Autodesk Inventor part; units mm, degrees
ref_plane "Work Plane1" through (-2.8393, 0, 0) normal (0, 0, -1) x (-1, 0, 0)
ref_plane "Work Plane2" through (0, 0, 4.58) normal (1, 0, 0) x (0, 0, -1)
ref_plane "Work Plane3" through (0, 45, 0) normal (0, 1, 0) x (1, 0, 0)
sketch "Sketch1" plane through (0, 0, 0) normal (0, 1, 0) x (-1, 0, 0)
  circle A0 centre (0, 0) radius 2.1
  line L0 (10, 10) -> (-10, 10) construction
  line L1 (-10, 10) -> (-10, -10) construction
  line L2 (-10, -10) -> (10, -10)
  line L3 (10, -10) -> (10, 10) construction
  line L4 (10, 10) -> (-10, -10) construction
  line L5 (-10, 10) -> (10, -10) construction
  line L6 (8.2, 10) -> (8.2, -10) construction
  line L7 (3.9, 10) -> (3.9, -10) construction
  line L8 (8.2, 3.125) -> (8.2, -3.125) construction
  line L9 (10, 4.58) -> (10, -4.58) construction
  line L10 (8.2, 5.5) -> (8.2, -5.5) construction
  line L11 (3.3697, 4.4303) -> (4.4303, 3.3697) construction
  line L12 (10, 10) -> (10, 4.58)
  line L13 (10, 4.58) -> (8.545, 3.125)
  line L14 (8.545, 3.125) -> (8.2, 3.125)
  line L15 (8.2, 3.125) -> (8.2, 5.5)
  line L16 (14, 0) -> (-14, 0) construction
  line L17 (8.2, 5.5) -> (6.5607, 5.5)
  line L18 (6.5607, 5.5) -> (3.9, 2.8393)
  line L19 (3.9, 2.8393) -> (3.9, 0)
  line L20 (10, -10) -> (10, -4.58)
  line L21 (10, -4.58) -> (8.545, -3.125)
  line L22 (8.545, -3.125) -> (8.2, -3.125)
  line L23 (8.2, -3.125) -> (8.2, -5.5)
  line L24 (8.2, -5.5) -> (6.5607, -5.5)
  line L25 (6.5607, -5.5) -> (3.9, -2.8393)
  line L26 (3.9, -2.8393) -> (3.9, 0)
  line L27 (-10, 10) -> (-4.58, 10)
  line L28 (-4.58, 10) -> (-3.125, 8.545)
  line L29 (-3.125, 8.2) -> (-5.5, 8.2)
  line L30 (-5.5, 8.2) -> (-5.5, 6.5607)
  line L31 (-5.5, 6.5607) -> (-2.8393, 3.9)
  line L32 (-2.8393, 3.9) -> (0, 3.9)
  line L33 (2.8393, 3.9) -> (0, 3.9)
  line L34 (5.5, 6.5607) -> (2.8393, 3.9)
  line L35 (5.5, 8.2) -> (5.5, 6.5607)
  line L36 (3.125, 8.2) -> (5.5, 8.2)
  line L37 (3.125, 8.545) -> (3.125, 8.2)
  line L38 (4.58, 10) -> (3.125, 8.545)
  line L39 (-3.125, 8.545) -> (-3.125, 8.2)
  line L40 (10, 10) -> (4.58, 10)
  line L41 (-10, -10) -> (-10, -4.58)
  line L42 (-10, -4.58) -> (-8.545, -3.125)
  line L43 (-8.2, -3.125) -> (-8.2, -5.5)
  line L44 (-8.2, -5.5) -> (-6.5607, -5.5)
  line L45 (-6.5607, -5.5) -> (-3.9, -2.8393)
  line L46 (-3.9, -2.8393) -> (-3.9, 0)
  line L47 (-3.9, 2.8393) -> (-3.9, 0)
  line L48 (-6.5607, 5.5) -> (-3.9, 2.8393)
  line L49 (-8.2, 5.5) -> (-6.5607, 5.5)
  line L50 (-8.2, 3.125) -> (-8.2, 5.5)
  line L51 (-8.545, 3.125) -> (-8.2, 3.125)
  line L52 (-10, 4.58) -> (-8.545, 3.125)
  line L53 (-8.545, -3.125) -> (-8.2, -3.125)
  line L54 (-10, 10) -> (-10, 4.58)
  line L55 (10, -10) -> (4.58, -10) construction
  line L56 (4.58, -10) -> (3.125, -8.545)
  line L57 (3.125, -8.2) -> (5.5, -8.2)
  line L58 (5.5, -8.2) -> (5.5, -6.5607)
  line L59 (5.5, -6.5607) -> (2.8393, -3.9)
  line L60 (2.8393, -3.9) -> (0, -3.9)
  line L61 (-2.8393, -3.9) -> (0, -3.9)
  line L62 (-5.5, -6.5607) -> (-2.8393, -3.9)
  line L63 (-5.5, -8.2) -> (-5.5, -6.5607)
  line L64 (-3.125, -8.2) -> (-5.5, -8.2)
  line L65 (-3.125, -8.545) -> (-3.125, -8.2)
  line L66 (-4.58, -10) -> (-3.125, -8.545)
  line L67 (3.125, -8.545) -> (3.125, -8.2)
  line L68 (-10, -10) -> (-4.58, -10) construction
  line L69 (5.5, -6.5607) -> (6.2393, -7.3)
  line L70 (6.2393, -7.3) -> (8.2, -7.3)
  line L71 (0, -10) -> (0, -9) construction
  line L72 (-5.5, -6.5607) -> (-6.2393, -7.3)
  line L73 (-6.2393, -7.3) -> (-8.2, -7.3)
  line L74 (8.2, -7.3) -> (8.2, -10)
  line L75 (-8.2, -7.3) -> (-8.2, -10)
  point P0 (10, 0)
  point P1 (8.2, 0)
  point P2 (3.9, 3.9)
  point P3 (-3.3697, 4.4303)
  point P4 (-4.4303, -3.3697)
  point P5 (3.3697, -4.4303)
  dimension "d0" = 4.2
  dimension "d1" = 20
  dimension "d2" = 20
  dimension "d3" = 1.8
  dimension "d4" = 4.3
  dimension "d5" = 6.25
  dimension "d6" = 9.16
  dimension "d7" = 11
  dimension "d8" = 1.5
  dimension "d9" = 45
  dimension "d12" = 360
  dimension "d17" = 1.8
  dimension "d18" = 1
extrude "Extrusion1" add sketch "Sketch1" along normal blind 90 contours L41 L42 L53 L43 L44 L45 L46 L47 L48 L49 L50 L51 L52 L54 L27 L28 L39 L29 L30 L31 L32 L33 L34 L35 L36 L37 L38 L40 L12 L13 L14 L15 L17 L18 L19 L26 L25 L24 L23 L22 L21 L20 L2 L74 L70 L69 L59 L60 L61 L62 L72 L73 L75 | L75 L73 L72 L63 L64 L65 L66 L2 | L56 L67 L57 L58 L69 L70 L74 L2
ref_plane "Work Plane1" through (-2.8393, 0, 0) normal (0, 0, -1) x (-1, 0, 0)
ref_plane "Work Plane2" through (0, 0, 4.58) normal (1, 0, 0) x (0, 0, -1)
ref_plane "Work Plane3" through (0, 45, 0) normal (0, 1, 0) x (1, 0, 0)
ref_plane "Work Plane4" through (-4.58, 0, 0) normal (0, 0, 1) x (1, 0, 0)
ref_plane "Work Plane5" through (0, 45, 0) normal (0, -1, 0) x (1, 0, 0)
ref_plane "Work Plane6" through (10, 0, 0) normal (0, 0, 1) x (1, 0, 0)
ref_plane "Work Plane7" through (0, 0, 4.58) normal (1, 0, 0) x (0, 0, -1)
properties part number "VSLOT 2020 Extrusion Mini" material "Aluminum 6061"
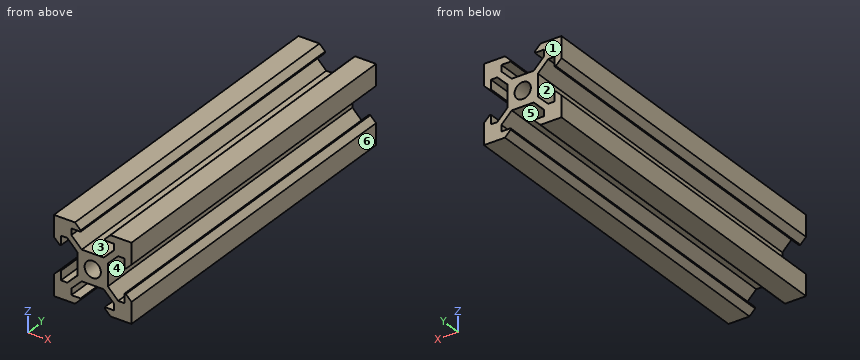
Geometry: final body of the model. Coordinates: model frame, mm. Face numbers are marked on the shaded views. A direction names the side the tool comes from. Coordinates: 2 decimals unless noted, no trailing zeros. Order: outer loops, then holes, each group sorted by start corner. A loop starts at its lowest first (then second) coordinate and runs counter-clockwise, first axis right, second up. Notation, with made-up numbers: (29.5, 6.25) -> (82.5, 6.25) arc R36 cw to (82.5, 40.25) -> close; hole circle Ø11 at (6, 50.5). An arc over 180 degrees is marked (long way). Use CSV: the item, a comma, the result in double quotes.
1) Section B-B on z = 0. Output: boundary loops of the cut face in (x, y), then the cut area to 3 significant figures.
Findings:
outline,"(-3.9, 0) -> (-2.1, 0) -> (-2.1, 90) -> (-3.9, 90) -> close; (2.1, 0) -> (3.9, 0) -> (3.9, 90) -> (2.1, 90) -> close"
area,"324 mm^2"
2) Mould query, pull axis Z, two halves, no side actions, for the marked faces 1, 2 and 3. Classes: +Z half, -Z half, draft (parallel to the pull), parting line (faces both ways), or undercut.
Findings:
face 1,"draft"
face 2,"undercut"
face 3,"+Z half"
3) Pin query (flat end, axial travel): pin 1 Ø3 at (x, y) = (1.5, 25.5) entering from -Z; pin 2 Ø1.9 at (y, z) = (65, 3.5) entering from -X; pin 3 Ø0.7 at (x, y) = (-4, 48.5) entering from -Z. Return the tip coordinate at first contact, or that it passes through.
Findings:
pin 1,"stops at z = -4.06"
pin 2,"stops at x = -9.87"
pin 3,"stops at z = -9.77"
4) Access query for the marked faces 4, 5 and 6. Directions: +Z, -Z, +X, -X, +Y, -Y. A direction counts if a zero-diameter tool reaches every point of the face in a straight line with its end or side. Return the directions, or none.
Findings:
face 4,"+X, +Y, -Y"
face 5,"-Z, +Y, -Y"
face 6,"+Z, -Z, +X, +Y, -Y"
5) Line query: line 1 (Z direction, x = 7.75, y = 72.5); line 2 (X direction, y = 64, z = -4.75); line 3 (X direction, y = 75, z = -0.25). Output: solid intervals per line, ascending.
Findings:
line 1,"z = -10 to -5.5, 5.5 to 10"
line 2,"x = -10 to -8.2, -5.81 to -3.69, 3.69 to 5.81, 8.2 to 10"
line 3,"x = -3.9 to -2.09, 2.09 to 3.9"
6) Section A-A on x = 0. Output: boundary loops of the cut face in (y, z).
Findings:
outline,"(0, -3.9) -> (90, -3.9) -> (90, -2.1) -> (0, -2.1) -> close; (0, 2.1) -> (90, 2.1) -> (90, 3.9) -> (0, 3.9) -> close"
